```python
from build123d import *

# Parameters (mm, degrees)
BOSS_EXTRUDE1_DEPTH = 27
BOSS_EXTRUDE2_DEPTH = 14.3
CUT_EXTRUDE1_DEPTH  = 6
SKETCH4_W           = 6
SKETCH4_H           = 44.518768508
CUT_EXTRUDE2_DEPTH  = 66


with BuildPart() as part:
    # Sketch1 → Boss-Extrude1 (new body)
    with BuildSketch(Plane.XY):
        Polygon((0, 0), (-6.81828161, 0), (-6.81828161, 76.4), (-0.81828161, 76.4), (-0.81828161, 6), (0, 6), align=None)
    extrude(amount=BOSS_EXTRUDE1_DEPTH)

    # Sketch2 → Boss-Extrude2 (add)
    with BuildSketch(Plane(origin=(0, 0, 0), x_dir=(-1, 0, 0), z_dir=(0, 0, -1))):
        Polygon((0.81828161, 6), (0, 6), (0, 0), (6.81828161, 0), (6.81828161, 76.4), (0.81828161, 76.4), align=None)
    extrude(amount=BOSS_EXTRUDE2_DEPTH)

    # Sketch3 → Cut-Extrude1 (cut)
    with BuildSketch(Plane(origin=(0, 6, 0), x_dir=(1, 0, 0), z_dir=(0, 1, 0))):
        with BuildLine():
            Line((8.68171839, -2.04396728), (-3.41828161, -2.04396728))
            ThreePointArc((-3.41828161, -2.04396728), (-6.37431433, -5), (-3.41828161, -7.95603272))
            Line((-3.41828161, -7.95603272), (8.68171839, -7.95603272))
            ThreePointArc((8.68171839, -7.95603272), (11.63775111, -5), (8.68171839, -2.04396728))
        make_face()
        with BuildLine():
            Line((8.68171839, -19.04396728), (-3.41828161, -19.04396728))
            ThreePointArc((-3.41828161, -19.04396728), (-6.37431433, -22), (-3.41828161, -24.95603272))
            Line((-3.41828161, -24.95603272), (8.68171839, -24.95603272))
            ThreePointArc((8.68171839, -24.95603272), (11.63775111, -22), (8.68171839, -19.04396728))
        make_face()
    extrude(amount=-CUT_EXTRUDE1_DEPTH, mode=Mode.SUBTRACT)

    # Sketch4 → Cut-Extrude2 (cut)
    with BuildSketch(Plane(origin=(0, 0, -14.3), x_dir=(-1, 0, 0), z_dir=(0, 0, -1))):
        with Locations((3.81828161, 54.140615746)):
            Rectangle(SKETCH4_W, SKETCH4_H)
    extrude(amount=-CUT_EXTRUDE2_DEPTH, mode=Mode.SUBTRACT)


solid = part.part
```
Check sheet for the modelled part. Datum: model origin and axes. Units: mm. A direction names the side the tool comes from. Give positions to 0.01 mm unless a question says otherwise; leave off trailing zeros. Order: outer loops, then holes, each group sorted by start corner. A loop starts at its lowest first (then second) coordinate and runs counter-clockwise, first axis right, second up. Notation, with made-up numbers: M 38,12.25 L 67,12.25 A20 ccw 67,30.25 Z; hole C -25.5,82 d3. An arc over 180 degrees is marked long. Answer in a Markdown table with one row per item.
1) Cross-section at C-C, the plane x = -1.75. Enter the section's corners in (y, z).
Filled sheet:
| item | result |
|---|---|
| outline | M 0,-14.3 L 31.88,-14.3 L 31.88,27 L 0,27 L 0,24.96 L 6,24.96 L 6,19.04 L 0,19.04 L 0,7.96 L 6,7.96 L 6,2.04 L 0,2.04 Z |
2) Cross-section at A-A, the plane y = 3. Enter the section's corners in (x, z), plus the area to 3 significant figures.
Filled sheet:
| item | result |
|---|---|
| outline | M -6.82,-14.3 L 0,-14.3 L 0,2.04 L -3.42,2.04 A2.96 cw -3.42,7.96 L 0,7.96 L 0,19.04 L -3.42,19.04 A2.96 cw -3.42,24.96 L 0,24.96 L 0,27 L -6.82,27 Z |
| area | 214 mm2 |
3) Cross-section at D-D, the plane z = -10. Enter the section's corners in (x, y).
Filled sheet:
| item | result |
|---|---|
| outline | M -6.82,0 L 0,0 L 0,6 L -0.82,6 L -0.82,31.88 L -6.82,31.88 Z |
4) Thickness scan on L1, parallel to Z at x = -1.75, y = 2.5; L2, parallel to Y at x = -3, z = 19.5; L3, parallel to X at y = 12.5, z = 10.5. Record the ranges inside material, lowest first. Write a range as [from, to].
Filled sheet:
| item | result |
|---|---|
| L1 | z = [-14.3, 2.04], [7.96, 19.04], [24.96, 27] |
| L2 | y = [6, 31.88] |
| L3 | x = [-6.82, -0.82] |
5) Cross-section at B-B, the plane z = 22. Enter the section's corners in (x, y).
Filled sheet:
| item | result |
|---|---|
| outline | M -6.82,0 L -6.37,0 L -6.37,6 L -0.82,6 L -0.82,31.88 L -6.82,31.88 Z |
6) Gauge pin test, flat ends, axial feed: P1, Ø1.7, axis at x = -3, z = 6.5, coming from the -Y side; P2, Ø13, axis at y = 16.5, z = -3.5, coming from the +X side. Record the tip position at first contact, or that the pin passes through.
Filled sheet:
| item | result |
|---|---|
| P1 | stops at y = 6 |
| P2 | stops at x = -0.82 |
7) Access from +Z, -Z, +X, -X, +Y, -Y to the whole of each face (thin tool, end or side, straight path). Record for faces 1 (the flat face through (-6, 0, 7)), 2 (the flat face through (-0.4, 6, 13.6)), 3 (the flat face through (-2, 3, 24.956)).
Filled sheet:
| item | result |
|---|---|
| face 1 | +Z, -Z, +X, -X, -Y |
| face 2 | +Z, -Z, +X, +Y |
| face 3 | +X, -Y |
8) Release check for a two-part mould opening along Z. For faces 4 (the flat face through (-0.818, 19, 7)), 5 (the flat face through (-3, 16, 27)), 6 (the flat face through (-4, 6, 22)), 7 (the flat face through (-2, 3, 19.044)) record: +Z half, -Z half, draft (parallel to the pull), parting line (faces both ways), or undercut.
Filled sheet:
| item | result |
|---|---|
| face 4 | draft |
| face 5 | +Z half |
| face 6 | undercut |
| face 7 | undercut |
